Study the drawing (mm; zero at the part's minimum x, y, z) and answer. A direction names the side the tool comes from. Give positions to 0.01 mm unless a question says otherwise; leave off trailing zeros. Order: outer loops, then holes, each group sorted by start corner. A loop starts at its lowest first (then second) coordinate and runs counter-clockwise, first axis right, second up. Notation, with made-up numbers: (-38.5, 30.25) - (-8.5, 30.25) arc R19 cw to (-8.5, 55.25) - close; hole circle Ø6 at (74, 49.5). An arc over 180 degrees is marked (long way). Return JSON: item names as keys, results as strings.
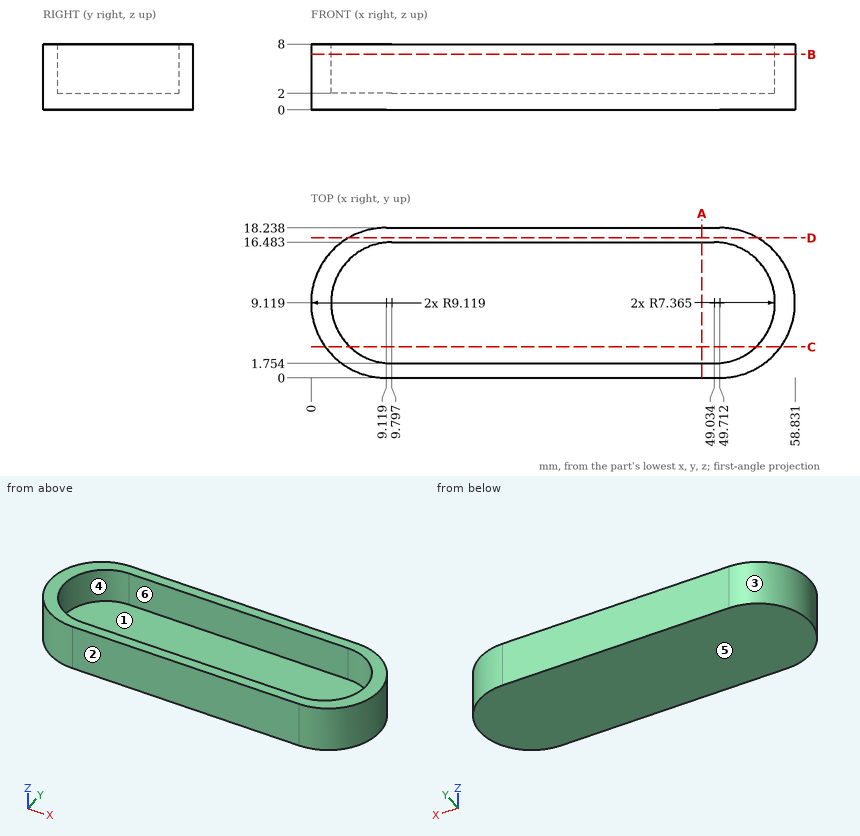
Q1. Consider L1, parallel to Y at x = 14, z = 7 (1 decimal); L2, parallel to Z at x = 26, y = 11.75; L3, parallel to X at y = 4.75, z = 6 (1 decimal). Determine where each line is inside the solid, lowest interval first.
Values:
{"L1": "y = 0 to 1.8, 16.5 to 18.2", "L2": "z = 0 to 2", "L3": "x = 1.1 to 3.9, 55 to 57.7"}
Q2. A cutting plane is placed at C-C (y = 3.75). Write down the section's boundary in (x, z) (1 decimal).
Values:
{"outline": "(1.7, 0) - (57.1, 0) - (57.1, 8) - (54.1, 8) - (54.1, 2) - (4.8, 2) - (4.8, 8) - (1.7, 8) - close"}
Q3. A cutting plane is placed at A-A (x = 47.5). Write down the section's boundary in (y, z) (1 decimal).
Values:
{"outline": "(0, 0) - (18.2, 0) - (18.2, 8) - (16.5, 8) - (16.5, 2) - (1.8, 2) - (1.8, 8) - (0, 8) - close"}
Q4. Determine the mould class of the marked faces 3, 4, 5 and 6 for opening direction X: released by +X, released by -X, zero draft, split by the parting line, or undercut.
Values:
{"face 3": "released by -X", "face 4": "undercut", "face 5": "zero draft", "face 6": "undercut"}
Q5. Given pin 1 (10 mm diameter, centred on x = 30.5, y = 9, fed in from -Z); pin 2 (4 mm diameter, centred on y = 3, z = 1, fed in from +X); pin 3 (6 mm diameter, centred on x = 19.5, y = 7, fed in from +Z), each flat-ended and moving along its own axis, determine where each tip first touches the part or whether it passes through.
Values:
{"pin 1": "stops at z = 0", "pin 2": "stops at x = 57.85", "pin 3": "stops at z = 2"}
Q6. A cutting plane is placed at B-B (z = 6.75). Write down the section's boundary in (x, y) (1 decimal).
Values:
{"outline": "(9.1, 0) - (49.7, 0) arc R9.1 ccw to (49.7, 18.2) - (9.1, 18.2) arc R9.1 ccw to start; hole (9.8, 1.8) - (49, 1.8) arc R7.4 ccw to (49, 16.5) - (9.8, 16.5) arc R7.4 ccw to start"}
Q7. A cutting plane is placed at D-D (y = 17). Write down the section's boundary in (x, z), and give its area (3 significant figures).
Values:
{"outline": "(4.53, 0) - (54.3, 0) - (54.3, 8) - (4.53, 8) - close", "area": "398 mm²"}
Q8. For the marked faces 1 and 2, determine the directions among +Z, -Z, +X, -X, +Y, -Y from which every point of the face is accessible in a straight line to the end or side of a thin tool.
Values:
{"face 1": "+Z", "face 2": "+Z, -Z, +X, -X, -Y"}
